Source: CAD feature listing. Evaluate the final solid. Frame: model axes, mm. A direction names the side the tool comes from. Coordinates: 2 decimals unless noted, no trailing zeros. Loops run counter-clockwise (first coordinate to the right, second up) from the corner with the lowest first, then second, coordinate; pieces in that order, holes last.
Item 1: Section query D-D, the plane z = 76.5. Return the cut outline in (x, y), then the cut area to 3 significant figures.
Item 2: Section query B-B, the plane z = 22. Return the cut outline in (x, y).
Item 3: Line query: probe 1 along X at (y, z) = (-1, 7); probe 2 along Z at (x, y) = (-117, -4.75); probe 3 along Y at (x, z) = (-116.5, 88.5). Output: solid intervals per line, ascending.
Item 4: Pull-direction query (X, two-part tool) for faces 6 (the flat face through (-106.376, 0, 110)), 7 (the flat face through (-102.934, 0.126, 117.635)), 8 (the flat face through (-120.25, 0.13, 2.08)); classes: +X half, -X half, draft (parallel to the pull), parting line (faces both ways), or undercut.
Item 5: Section query C-C, the plane z = 91. Return the cut outline in (x, y).
Item 6: Pin query (flat end, axial travel): pin 1 Ø10 at (x, z) = (-122.5, 86.5) entering from +Y; pin 2 Ø5 at (y, z) = (-3.5, 24) entering from +X; pin 3 Ø13 at (x, z) = (-118, 35.5) entering from -Y; pin 4 Ø3 at (x, z) = (-126.87, 83.59) entering from -Y. Return the tip coordinate at first contact, or that it passes through.
Item 7: Section query A-A, the plane x = -116. Return the cut outline in (y, z), then the cut area to 3 significant figures.
Item 8: Reachability of faces 1 (the flat face through (-100.858, 0.126, 76.596)), 2 (the cylindrical face through (-116.026, 8.493, 66.024)), 3 (the flat face through (-126.9, 0.13, 77.75)), 4 (the flat face through (-121, -8, 40)), 5 (the flat face through (-117.906, 0, 124)) from +Z, -Z, +X, -X, +Y, -Y: full face, straight path, thin tool, end or side. Return the list, or none.
```python
from build123d import *

# Parameters (mm, degrees)
BOSS_EXTRUDE2_DEPTH   = 9
FILLET3_R             = 4
FILLET4_R             = 4
FILLET5_R             = 4
BOSS_EXTRUDE3_DEPTH   = 18
LPATTERN1_COUNT       = 6
LPATTERN1_PITCH       = 6
MIRROR1_START         = -8.124245185
MIRROR1_OUTLINE_R     = 1.5
MIRROR1_DEPTH         = 12.777246129
MIRROR1_START_2       = -9
MIRROR1_2_OUTLINE_R   = 1.5
MIRROR1_2_DEPTH       = 18
MIRROR1_3_DEPTH       = 1
MIRROR1_START_3       = 8
MIRROR1_4_DEPTH       = 1
MIRROR1_START_4       = -11
MIRROR1_5_OUTLINE_R   = 1.75
MIRROR1_5_DEPTH       = 22
MIRROR1_START_5       = -12
MIRROR1_6_OUTLINE_R   = 1.75
MIRROR1_6_OUTLINE_R_2 = 1.55
MIRROR1_6_DEPTH       = 24
MIRROR1_START_6       = -136.757331166
MIRROR1_7_DEPTH       = 7.999999999


with BuildPart() as part:
    # Sketch2 → Boss-Extrude2 (new, symmetric)
    with BuildSketch(Plane(origin=(0, 0, 0), x_dir=(1, 0, 0), z_dir=(0, 1, 0))):
        Polygon((-131.994556455, -4.071203001), (-120.287458623, -73.085287508), (-107.994556455, -71), (-107.994556455, 0), align=None)
        with BuildLine():
            ThreePointArc((-106.180430892, -65.996333846), (-97.650502603, -65.078471315), (-96.922675808, -73.626711859))
            Line((-96.922675808, -73.626711859), (-104.905552704, -79.64947505))
            Line((-104.905552704, -79.64947505), (-104.905552704, -129.64947505))
            Line((-104.905552704, -129.64947505), (-117.905552704, -129.64947505))
            Line((-117.905552704, -129.64947505), (-117.905552704, -122.64947505))
            Line((-117.905552704, -122.64947505), (-122.994556455, -92.64947505))
            Line((-122.994556455, -92.64947505), (-132.520871847, -83.803610759))
            Line((-132.520871847, -83.803610759), (-122.994556455, -73.544501876))
            Line((-122.994556455, -73.544501876), (-107.994556455, -71))
            Line((-107.994556455, -71), (-107.755356075, -71))
            Line((-107.755356075, -71), (-106.180430892, -65.996333846))
        make_face()
    extrude(amount=BOSS_EXTRUDE2_DEPTH, both=True)

    # Fillet3
    fillet3_edges = [part.edges().sort_by_distance(p)[0] for p in [
        (-131.994556455, 0, 4.071203001),
        (-107.994556455, 0, 0),
    ]]
    fillet(fillet3_edges, radius=FILLET3_R)

    # Fillet4
    fillet4_edges = [part.edges().sort_by_distance(p)[0] for p in [
        (-132.520871847, 0, 83.803610759),
        (-122.994556455, 0, 73.544501876),
    ]]
    fillet(fillet4_edges, radius=FILLET4_R)

    # Fillet5
    fillet5_edges = [part.edges().sort_by_distance(p)[0] for p in [
        (-117.905552704, 0, 129.64947505),
    ]]
    fillet(fillet5_edges, radius=FILLET5_R)

    # Sketch4 → Boss-Extrude3 (add)
    with BuildSketch(Plane(origin=(0, 9, 0), x_dir=(1, 0, 0), z_dir=(0, 1, 0))):
        Polygon((-104.905552704, -126.64947505), (-104.905552704, -122.64947505), (-100.905552704, -124.64947505), align=None)
    boss_extrude3 = extrude(amount=-BOSS_EXTRUDE3_DEPTH)

    # LPattern1: Boss-Extrude3 ×6
    with Locations(*[(0, 0, -i * LPATTERN1_PITCH) for i in range(1, LPATTERN1_COUNT)]):
        add(boss_extrude3)

    # Mirror1: read off the stored shape, not the designer's step
    # Mirror1 outline → Mirror1 (cut)
    with BuildSketch(Plane(origin=(0, 0, 0), x_dir=(1, 0, 0), z_dir=(0, 1, 0)).offset(MIRROR1_START)):
        Polygon((-106.375961974, -96.859639276), (-121.375961974, -96.859639276), (-119.951756879, -99.233314435), (-121.823846672, -99.550883501), (-118.741773978, -117.719897586), (-110.854450034, -116.381943548), (-111.324238264, -113.612512127), (-106.375961974, -121.859639276), align=None)
        with Locations((-127.381917465, -7.345887954)):
            Circle(MIRROR1_OUTLINE_R)
    extrude(amount=MIRROR1_DEPTH, mode=Mode.SUBTRACT)

    # Mirror1 2 outline → Mirror1 2 (cut)
    with BuildSketch(Plane(origin=(0, 0, 0), x_dir=(1, 0, 0), z_dir=(0, 1, 0)).offset(MIRROR1_START_2)):
        Polygon((-106.375961974, -96.859639276), (-121.375961974, -96.859639276), (-106.375961974, -121.859639276), align=None)
        with Locations((-127.381917465, -7.345887954)):
            Circle(MIRROR1_2_OUTLINE_R)
    extrude(amount=MIRROR1_2_DEPTH, mode=Mode.SUBTRACT)

    # Mirror1 3 outline → Mirror1 3 (cut)
    with BuildSketch(Plane(origin=(0, 0, 0), x_dir=(1, 0, 0), z_dir=(0, 1, 0)).offset(MIRROR1_START_2)):
        with BuildLine():
            Line((-114.481804476, -63.909695389), (-122.650561904, -15.020919875))
            ThreePointArc((-122.650561904, -15.020919875), (-124.758454252, -13.516588893), (-126.262785233, -15.624481241))
            Line((-126.262785233, -15.624481241), (-118.094027806, -64.513256756))
            ThreePointArc((-118.094027806, -64.513256756), (-115.986135457, -66.017587738), (-114.481804476, -63.909695389))
        make_face()
    extrude(amount=MIRROR1_3_DEPTH, mode=Mode.SUBTRACT)

    # Mirror1 4 outline → Mirror1 4 (cut)
    with BuildSketch(Plane(origin=(0, 0, 0), x_dir=(1, 0, 0), z_dir=(0, 1, 0)).offset(MIRROR1_START_3)):
        with BuildLine():
            Line((-114.481804476, -63.909695389), (-122.650561904, -15.020919875))
            ThreePointArc((-122.650561904, -15.020919875), (-124.758454252, -13.516588893), (-126.262785233, -15.624481241))
            Line((-126.262785233, -15.624481241), (-118.094027806, -64.513256756))
            ThreePointArc((-118.094027806, -64.513256756), (-115.986135457, -66.017587738), (-114.481804476, -63.909695389))
        make_face()
    extrude(amount=MIRROR1_4_DEPTH, mode=Mode.SUBTRACT)

    # Mirror1 5 outline → Mirror1 5 (add)
    with BuildSketch(Plane(origin=(0, 0, 0), x_dir=(1, 0, 0), z_dir=(0, 1, 0)).offset(MIRROR1_START_4)):
        with Locations((-126.867893483, -83.59424119)):
            Circle(MIRROR1_5_OUTLINE_R)
        with Locations((-101.466636513, -69.708495286)):
            Circle(MIRROR1_5_OUTLINE_R)
    extrude(amount=MIRROR1_5_DEPTH)

    # Mirror1 6 outline → Mirror1 6 (add)
    # profile 1 of 2: a face of its own
    with BuildSketch(Plane(origin=(0, 0, 0), x_dir=(1, 0, 0), z_dir=(0, 1, 0)).offset(MIRROR1_START_5)):
        with Locations((-126.867893483, -83.59424119)):
            Circle(MIRROR1_6_OUTLINE_R)
        with Locations((-126.867893483, -83.59424119)):
            Circle(MIRROR1_6_OUTLINE_R_2, mode=Mode.SUBTRACT)
    # profile 2 of 2: a face of its own
    with BuildSketch(Plane(origin=(0, 0, 0), x_dir=(1, 0, 0), z_dir=(0, 1, 0)).offset(MIRROR1_START_5)):
        with Locations((-101.466636513, -69.708495286)):
            Circle(MIRROR1_6_OUTLINE_R)
        with Locations((-101.466636513, -69.708495286)):
            Circle(MIRROR1_6_OUTLINE_R_2, mode=Mode.SUBTRACT)
    extrude(amount=MIRROR1_6_DEPTH)

    # Mirror1 7 outline → Mirror1 7 (cut)
    with BuildSketch(Plane(origin=(0, 0, 0), x_dir=(0, 1, 0), z_dir=(0.9859154929577465, 0, -0.1672442547470129)).offset(MIRROR1_START_6)):
        Polygon((4.653000944, 77.774419934), (7.4664805, 77.774419934), (4.653000944, 96.202991363), align=None)
        Polygon((-8.124245185, 77.774419934), (-8.124245185, 96.202991363), (-8.855207199, 96.202991363), align=None)
    extrude(amount=MIRROR1_7_DEPTH, mode=Mode.SUBTRACT)


solid = part.part
```
Verdict:
1. outline: (-125.74, -9) - (-100.73, -9) - (-100.73, 9) - (-125.74, 9) - close
1. area: 450 mm2
2. outline: (-128.95, -9) - (-125.2, -9) - (-125.2, -8) - (-121.48, -8) - (-121.48, -9) - (-107.99, -9) - (-107.99, 9) - (-121.48, 9) - (-121.48, 8) - (-125.2, 8) - (-125.2, 9) - (-128.95, 9) - close
3. probe 1: x = -131.37 to -128.84, -125.92 to -107.99
3. probe 2: z = 1.53 to 96.86, 117.42 to 128.18
3. probe 3: y = -9 to 9
4. face 6: undercut
4. face 7: +X half
4. face 8: -X half
5. outline: (-124.77, -9) - (-104.91, -9) - (-104.91, 9) - (-124.77, 9) - close
6. pin 1: stops at y = 12
6. pin 2: stops at x = -107.99
6. pin 3: stops at y = -9
6. pin 4: stops at y = -11
7. outline: (-9, 1.36) - (9, 1.36) - (9, 54.82) - (8, 54.82) - (8, 66.02) - (9, 66.02) - (9, 96.86) - (-9, 96.86) - (-9, 66.02) - (-8, 66.02) - (-8, 54.82) - (-9, 54.82) - close; (-9, 105.82) - (-8.41, 105.82) - (-8.86, 117.25) - (4.65, 117.25) - (6.37, 105.82) - (9, 105.82) - (9, 129.06) - (-9, 129.06) - close
7. area: 1,950 mm2
8. face 1: +X, +Y, -Y
8. face 2: +Y
8. face 3: -X, +Y, -Y
8. face 4: -Y
8. face 5: +Z, -X, +Y, -Y
